Geometry: see drawing. Coordinates: mm, zero at the bounding-box minimum. Give positions to 0.01 mm unless a question says otherwise; leave off trailing zeros. Order: outer loops, then holes, each group sorted by start corner. A loop starts at its lowest first (then second) coordinate and runs counter-clockwise, first axis right, second up. Notation, with made-up numbers: M 56,25 L 115,25 A17 ccw 115,33 Z; hole C 17,35.5 d8. An arc over 180 degrees is marked long. Answer as a JSON object with one key per item and string values. Group by question number.
1. Section query B-B (y = 34). Output: boundary loops of the cut face in (x, z) (1 decimal), plus the area to 3 significant figures.
2. Section query C-C (z = 1.9). Output: boundary loops of the cut face in (x, y) (1 decimal), plus the area to 3 significant figures.
3. Section query A-A (x = 242). Output: boundary loops of the cut face in (y, z) (1 decimal).
4. Material intervals for L1, parallel to X at y = 148, z = 3.1 (1 decimal); L2, parallel to X at y = 176.5, z = 2.1 (1 decimal); L3, parallel to Y at x = 242, z = 2.75 (1 decimal), sorted ascending. Write a range as [from, to].
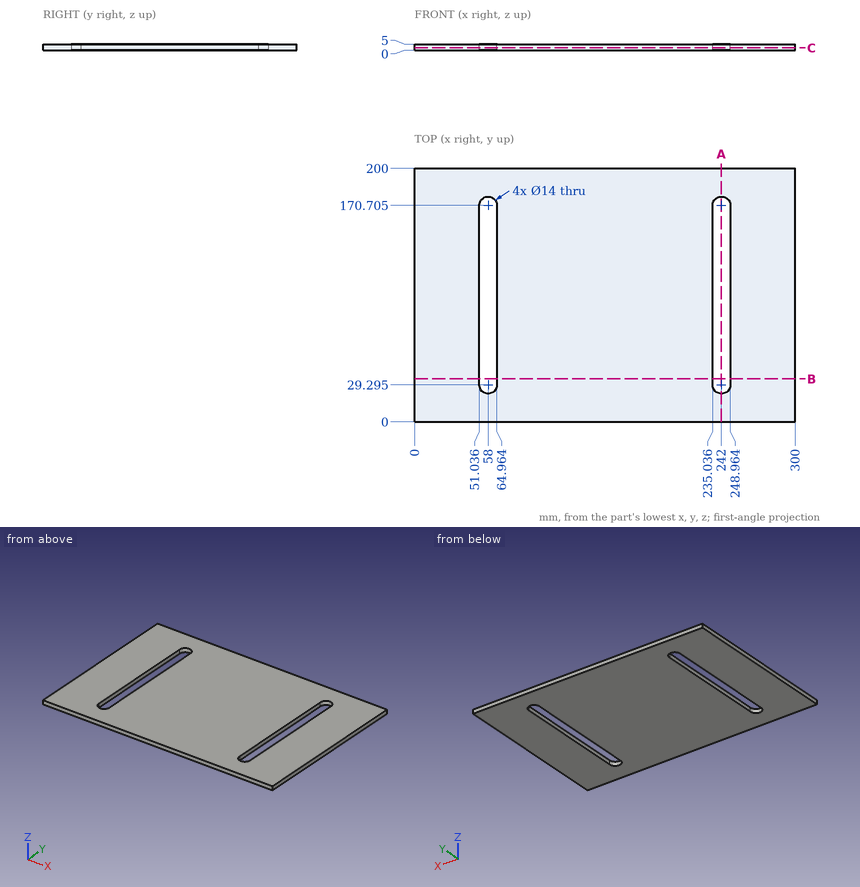
Answer sheet:
{
 "1": {"outline": "M 0,0 L 51,0 L 51,5 L 0,5 Z; M 65,0 L 235,0 L 235,5 L 65,5 Z; M 249,0 L 300,0 L 300,5 L 249,5 Z", "area": "1,360 mm^2"},
 "2": {"outline": "M 0,0 L 300,0 L 300,200 L 0,200 Z; hole M 51,30 A7 ccw long 65,30 L 65,170 A7 ccw long 51,170 Z; hole M 235,30 A7 ccw long 249,30 L 249,170 A7 ccw long 235,170 Z", "area": "55,800 mm^2"},
 "3": {"outline": "M 0,0 L 22.3,0 L 22.3,5 L 0,5 Z; M 177.7,0 L 200,0 L 200,5 L 177.7,5 Z"},
 "4": {"L1": "[0, 51], [65, 235], [249, 300]", "L2": "[0, 54.1], [61.9, 238.1], [245.9, 300]", "L3": "[0, 22.3], [177.7, 200]"}
}
